from build123d import *

# Parameters (mm, degrees)
SKETCH1_R           = 3.175
BOSS_EXTRUDE1_DEPTH = 3.175


with BuildPart() as part:
    # Sketch1 → Boss-Extrude1 (new body)
    with BuildSketch(Plane.XY):
        with BuildLine():
            Line((20.716035226, 7.9502), (0, 7.9502))
            ThreePointArc((0, 7.9502), (-7.9502, 0), (0, -7.9502))
            Line((0, -7.9502), (34.925, -7.9502))
            ThreePointArc((34.925, -7.9502), (40.310178716, -5.848549413), (42.84819283, -0.654748362))
            Line((42.84819283, -0.654748362), (47.452723337, 55.065258294))
            Line((47.452723337, 55.065258294), (47.625, 57.15))
            ThreePointArc((47.625, 57.15), (34.925, 69.85), (22.225, 57.15))
            Line((22.225, 57.15), (22.550500177, 54.29312161))
            Line((22.550500177, 54.29312161), (27.02521651, 15.019040407))
            ThreePointArc((27.02521651, 15.019040407), (25.453499558, 10.071851421), (20.716035226, 7.9502))
        make_face()
        Circle(SKETCH1_R, mode=Mode.SUBTRACT)
        with Locations((34.925, 0)):
            Circle(SKETCH1_R, mode=Mode.SUBTRACT)
        with Locations((34.925, 57.15)):
            Circle(SKETCH1_R, mode=Mode.SUBTRACT)
    extrude(amount=BOSS_EXTRUDE1_DEPTH)


solid = part.part
Can you work these out from the model? Positions are in its coordinate system, mm. A direction names the side the tool comes from. Coordinates: 2 decimals unless noted, no trailing zeros. Order: outer loops, then holes, each group sorted by start corner. A loop starts at its lowest first (then second) coordinate and runs counter-clockwise, first axis right, second up. Notation, with made-up numbers: M 67,17 L 73,17 A22 ccw 73,30 Z; hole C 22.5,-25.75 d7. An arc over 180 degrees is marked long. Answer as CSV lines item,"result".
(1) If we mould it in two halves opening along X, with no side actions, what happens to faces 1 (the cylindrical face through (37.953, 0.954, 1.565)), 2 (the cylindrical face through (40.249, -5.904, 1.565)), 3 (the cylindrical face through (-0.69, -3.1, 1.57)), 4 (the flat face through (32, 23, 3.175))? For each: released by +X, released by -X, zero draft, split by the parting line, or undercut.
Geometry check:
face 1,"undercut"
face 2,"released by +X"
face 3,"undercut"
face 4,"zero draft"
(2) Please list where these lines run through material, in increasing order: L1, parallel to Y at x = 0, z = 1.5 (3 decimals); L2, parallel to Y at x = 34, z = 1.85; L3, parallel to Y at x = 12.5, z = 2.95.
Geometry check:
L1,"-7.95 to -3.175, 3.175 to 7.95"
L2,"-7.95 to -3.04, 3.04 to 54.11, 60.19 to 69.82"
L3,"-7.95 to 7.95"
(3) On a 3-axis mill with a long thin cutter (end or side, diameter ignored), from which of +Z, -Z, +X, -X, +Y, -Y can I reach the whole of each face in a straight line? I mean faces 5 (the flat face through (17, -7.95, 2)), 6 (the flat face through (11, 7.95, 2)). Say none if no direction works.
Geometry check:
face 5,"+Z, -Z, +X, -X, -Y"
face 6,"+Z, -Z, -X, +Y"
(4) Suppose I cut it at B-B on x = 13.5. Please give me the cut outline in (y, z) (3 decimals), plus the area to 3 significant figures.
Geometry check:
outline,"M -7.95,0 L 7.95,0 L 7.95,3.175 L -7.95,3.175 Z"
area,"50.5 mm^2"
(5) Suppose I cut it at C-C on y = 41.5. Please give me the cut outline in (x, z) (3 decimals).
Geometry check:
outline,"M 24.008,0 L 46.332,0 L 46.332,3.175 L 24.008,3.175 Z"
(6) Suppose I cut it at A-A on z = 0.95. Count the separate pieces of the cut face and the enclosed holes in it, plus the area to 3 significant figures.
Geometry check:
separate pieces,"1"
enclosed holes,"3"
area,"1,950 mm^2"
(7) I'm going to push flat-ended pins straight in: pin 1 (5.5 mm diameter, centred on x = 34.925, y = 0, fed in from -Z); pin 2 (10 mm diameter, centred on x = 0, y = 0, fed in from +Z) (3 decimals); pin 3 (1 mm diameter, centred on y = 36.5, z = 1, fed in from -X); pin 4 (1 mm diameter, centred on y = 23, z = 2, fed in from +X). Where does each tip first touch, or does it pass through?
Geometry check:
pin 1,"through"
pin 2,"z = 3.175"
pin 3,"x = 24.52"
pin 4,"x = 44.84"
